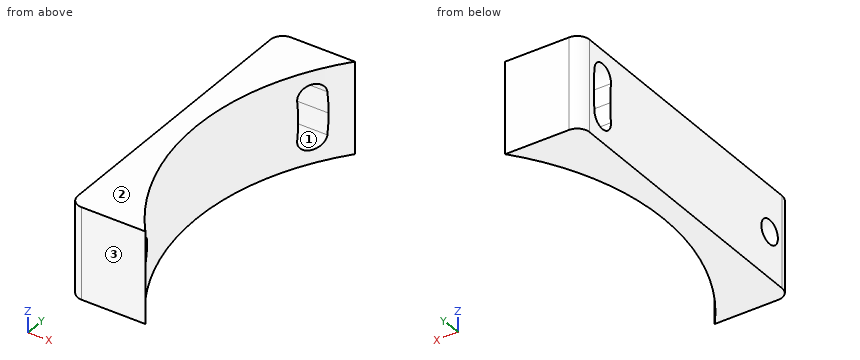
```python
from build123d import *

# Parameters (mm, degrees)
F1_DEPTH = 19.05
F4_D     = 5
F4_DEPTH = 15.7
F4_TIP   = 1.5021515476
F5_DEPTH = 25.4


with BuildPart() as f1:
    # F0 (on Top) → F1 (new body)
    with BuildSketch(Plane.XY):
        with BuildLine():
            ThreePointArc((-39.6557372898, -31.75), (-50.8, 0), (-39.6557372898, 31.75))
            Line((-39.6557372898, 31.75), (-52.8699082947, 31.75))
            ThreePointArc((-52.8699082947, 31.75), (-54.6659595189, 31.0060512242), (-55.4099082947, 29.21))
            Line((-55.4099082947, 29.21), (-55.4099082947, -29.21))
            ThreePointArc((-55.4099082947, -29.21), (-54.6659595189, -31.0060512242), (-52.8699082947, -31.75))
            Line((-52.8699082947, -31.75), (-39.6557372898, -31.75))
        make_face()
    extrude(amount=F1_DEPTH)

    # F4
    with Locations(Plane(origin=(-55.4099082947, 0, 0), x_dir=(0, -1, 0), z_dir=(-1, 0, 0))):
        with Locations((25.4, 9.525)):
            Hole(F4_D / 2, depth=F4_DEPTH)
            with Locations((0, 0, -(F4_DEPTH + F4_TIP / 2))):  # 118° drill point
                Cone(0, F4_D / 2, F4_TIP, mode=Mode.SUBTRACT)

    # F3 (on offset) → F5 (cut)
    with BuildSketch(Plane(origin=(-55.4099082947, 0, 0), x_dir=(0, -1, 0), z_dir=(-1, 0, 0))):
        with BuildLine():
            ThreePointArc((-27.7153407028, 13.9654662391), (-27.8542875294, 11.747165191), (-27.90063, 9.525))
            Line((-27.90063, 9.525), (-22.89937, 9.525))
            ThreePointArc((-22.89937, 9.525), (-22.8573758972, 11.538656851), (-22.7314666127, 13.5488121361))
            ThreePointArc((-22.7314666127, 13.5488121361), (-25.0150766063, 16.2490762326), (-27.7153407028, 13.9654662391))
        make_face()
        with BuildLine():
            Line((-22.89937, 9.525), (-27.90063, 9.525))
            ThreePointArc((-27.90063, 9.525), (-27.8542875294, 7.302834809), (-27.7153407028, 5.0845337609))
            ThreePointArc((-27.7153407028, 5.0845337609), (-25.0150766063, 2.8009237674), (-22.7314666127, 5.5011878639))
            ThreePointArc((-22.7314666127, 5.5011878639), (-22.8573758972, 7.511343149), (-22.89937, 9.525))
        make_face()
    extrude(amount=-F5_DEPTH, mode=Mode.SUBTRACT)


solid = f1.part
```
The listing builds one solid part. Answer for the finished solid, in the listing's coordinates (mm). Face numbers are marked on the shaded views. Coordinates: 2 decimals unless noted, no trailing zeros. Order: outer loops, then holes, each group sorted by start corner. A loop starts at its lowest first (then second) coordinate and runs counter-clockwise, first axis right, second up. Notation, with made-up numbers: M 43.5,81.25 L 97.5,81.25 A26 ccw 97.5,95.25 Z; hole C 74.5,-29.5 d1. An arc over 180 degrees is marked long. Answer as a JSON object with one key per item and string values. Group by question number.
1. Determine the mould class of the marked faces 1, 2 and 3 for opening direction Y: released by +Y, released by -Y, zero draft, split by the parting line, or undercut.
2. Straight lines are drawn through the part: line 1 (Z direction, x = -51.25, y = -25.4) (3 decimals); line 2 (Y direction, x = -46, z = 4); line 3 (Y direction, x = -52.75, z = 11). For each, find the intervals that lie inside material, in ascending order.
3. Section B-B on z = 15 is taken. Write down the section's boundary in (x, y), then the cut area to 3 significant figures.
4. Section C-C on y = -25.4 is taken. Write down the section's boundary in (x, z) (3 decimals).
5. Section A-A on x = -47.5 is taken. Write down the section's boundary in (y, z) (3 decimals).
6. Section D-D on y = -17 is taken. Write down the section's boundary in (x, z), then the cut area to 3 significant figures.
7. Flat-ended cylindrical pins translate along their axes: P1, Ø6.5, axis at y = -25.4, z = 9.525, coming from the +X side; P2, Ø1, axis at x = -44, y = 22, coming from the -Z side. Find the tip coordinate at first contact, or state that the pin passes through.
Values follow:
{
 "1": {"face 1": "undercut", "face 2": "zero draft", "face 3": "released by -Y"},
 "2": {"line 1": "0 to 7.025, 12.025 to 19.05", "line 2": "-31.75 to -21.56, 21.56 to 23.08, 27.36 to 31.75", "line 3": "-31.75 to -27.42, -23.38 to 22.88, 27.88 to 31.75"},
 "3": {"outline": "M -55.41,-29.21 A2.54 ccw -52.87,-31.75 L -39.66,-31.75 A50.8 cw -45.27,23.05 L -55.41,23.05 Z; M -55.41,27.39 L -42.78,27.39 A50.8 cw -39.66,31.75 L -52.87,31.75 A2.54 ccw -55.41,29.21 Z", "area": "465 mm2"},
 "4": {"outline": "M -55.41,0 L -43.994,0 L -43.994,7.025 L -55.41,7.025 Z; M -55.41,12.025 L -43.994,12.025 L -43.994,19.05 L -55.41,19.05 Z"},
 "5": {"outline": "M -31.75,0 L -18.011,0 L -18.011,19.05 L -31.75,19.05 Z; M 18.011,0 L 31.75,0 L 31.75,19.05 L 18.011,19.05 Z; hole C -25.4,9.525 d5; hole M 22.731,5.501 A2.501 ccw 27.715,5.085 A53.301 ccw 27.715,13.965 A2.501 ccw 22.731,13.549 A48.299 cw Z"},
 "6": {"outline": "M -55.41,0 L -47.87,0 L -47.87,19.05 L -55.41,19.05 Z", "area": "144 mm2"},
 "7": {"P1": "x = -41.95", "P2": "through"}
}
